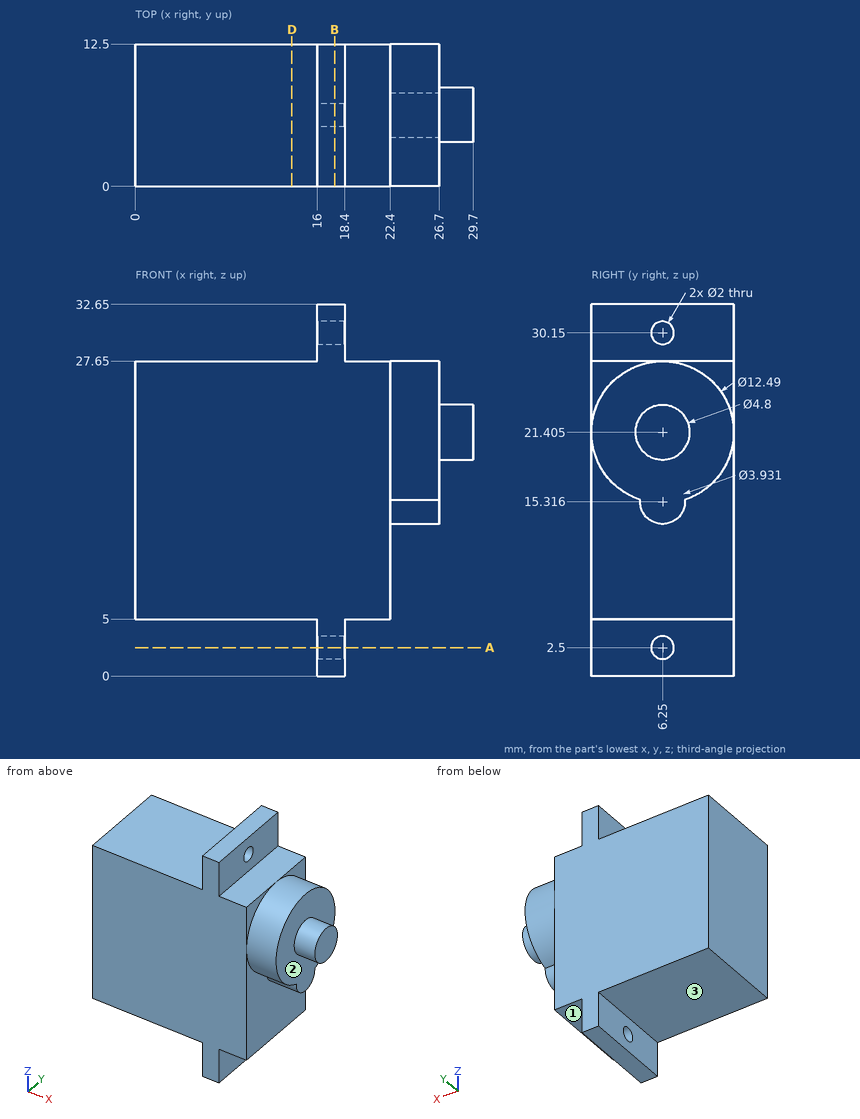
The figure shows three views and two pictorial views of one solid part (mm, origin at its lowest corner). Answer the questions. A direction names the side the tool comes from. Round coordinates to 2 decimals unless told otherwise and drop trailing zeros. Write each loop counter-clockwise with the first axis right and the second up, starting at its lowest first coordinate (ties: lowest second). Pieces come first, ordered by that corner, then holes. Notation, with made-up numbers: (65.5, -13) - (108.5, -13) arc R8 ccw to (108.5, -3) - close; hole circle Ø5 at (-17.5, 1.5). An arc over 180 degrees is marked (long way). Answer in a Markdown table with one row per item. Add a question column.
1. A cutting plane is placed at D-D, the plane x = 13.75. Determine the outline of the cut face in (y, z), and give its area (3 significant figures).
2. A cutting plane is placed at A-A, the plane z = 2.5. Determine the outline of the cut face in (x, y), and give its area (3 significant figures).
3. A cutting plane is placed at B-B, the plane x = 17.5. Determine the outline of the cut face in (y, z), and give its area (3 significant figures).
4. Find the intervals of material crossed by line 1 along Y through (x, z) = (16.7, 2.5); line 2 along Z through (x, y) = (3.25, 1.75); line 3 along X through (y, z) = (6.75, 1.5), in increasing order. Write a range as from..to.
5. For the marked faces 1, 2 and 3, determine the directions among +Z, -Z, +X, -X, +Y, -Y from which every point of the face is accessible in a straight line to the end or side of a thin tool.
6. Given pin 1 (4 mm diameter, centred on x = 4, y = 5, fed in from -Z); pin 2 (1.6 mm diameter, centred on y = 6.25, z = 2.5, fed in from -X); pin 3 (1.5 mm diameter, centred on y = 7.5, z = 3.5, fed in from +X); pin 4 (2.5 mm diameter, centred on y = 7, z = 2, fed in from -X), each flat-ended and moving along its own axis, determine where each tip first touches the part or whether it passes through.
Worked out:
| question | item | result |
|---|---|---|
| 1 | outline | (0, 5) - (12.5, 5) - (12.5, 27.65) - (0, 27.65) - close |
| 1 | area | 283 mm^2 |
| 2 | outline | (16, 0) - (18.4, 0) - (18.4, 5.25) - (16, 5.25) - close; (16, 7.25) - (18.4, 7.25) - (18.4, 12.5) - (16, 12.5) - close |
| 2 | area | 25.2 mm^2 |
| 3 | outline | (0, 0) - (12.5, 0) - (12.5, 32.65) - (0, 32.65) - close; hole circle Ø2 at (6.25, 2.5); hole circle Ø2 at (6.25, 30.15) |
| 3 | area | 402 mm^2 |
| 4 | line 1 | 0..5.25, 7.25..12.5 |
| 4 | line 2 | 5..27.65 |
| 4 | line 3 | 16..18.4 |
| 5 | face 1 | -Z, +X, +Y, -Y |
| 5 | face 2 | +X |
| 5 | face 3 | -Z, -X, +Y, -Y |
| 6 | pin 1 | z = 5 |
| 6 | pin 2 | through |
| 6 | pin 3 | x = 18.4 |
| 6 | pin 4 | x = 16 |
